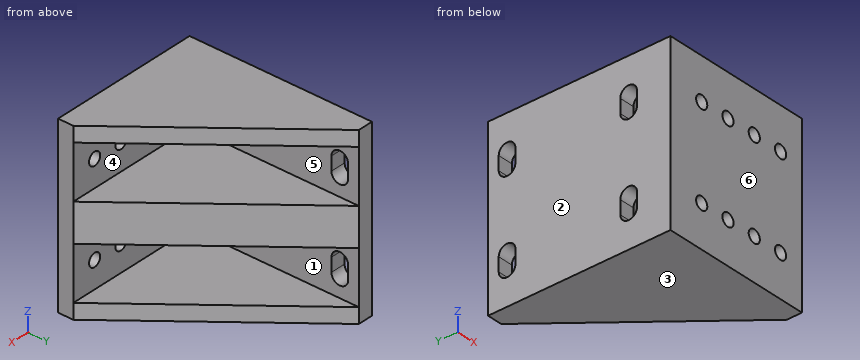
Autodesk Inventor part; units mm, degrees
ref_plane "YZ Plane" through (0, 0, 0) normal (1, 0, 0) x (0, 1, 0)
ref_plane "XZ Plane" through (0, 0, 0) normal (0, 1, 0) x (-1, 0, 0)
sketch "Sketch1" plane through (0, 0, 0) normal (0, 1, 0) x (-1, 0, 0)
  line L0 (-40, -23) -> (0, -23)
  line L1 (-40, 23) -> (0, 23)
  line L2 (0, 23) -> (0, -23)
  line L3 (-40, 23) -> (-40, -23)
  line L4 (-40, -12) -> (0, -12) construction
  line L5 (-40, 12) -> (0, 12) construction
  circle A0 centre (-9.5, 12) radius 1.7
  line L6 (-4, 23) -> (-4, -23) construction
  circle A1 centre (-17.5, 12) radius 1.7
  circle A2 centre (-25.5, 12) radius 1.7
  circle A3 centre (-33.5, 12) radius 1.7
  circle A4 centre (-9.5, -12) radius 1.7
  circle A5 centre (-17.5, -12) radius 1.7
  circle A6 centre (-25.5, -12) radius 1.7
  circle A7 centre (-33.5, -12) radius 1.7
  circle A8 centre (-9.5, 12) radius 3.5 construction
  line L7 (0, 19) -> (-40, 19) construction
  point P0 (0, 0)
  dimension "d5" = 46
  dimension "d6" = 23
  dimension "d7" = 40
  dimension "d8" = 0
  dimension "d9" = 12
  dimension "d10" = 12
  dimension "d11" = 3.4
  dimension "d12" = 4
  dimension "d13" = 9.5
  dimension "d16" = 8
  dimension "d19" = 24
  dimension "d22" = 7
  dimension "d23" = 4
extrude "Lift Attachment Plate" add sketch "Sketch1" along normal blind 4
sketch "Sketch2" plane through (0, 4, 0) normal (0, 1, 0) x (1, 0, 0)
  line L0 (0, 23) -> (0, -23)
  line L1 (40, 23) -> (0, 23)
  line L2 (0, -23) -> (4, -23)
  line L3 (4, -23) -> (4, 23)
  line L4 (4, 23) -> (0, 23)
  line L5 (0, 23) -> (0, -23)
  point P0 (0, 0)
  dimension "d26" = 4
extrude "Cross bar Attachment Plate" add sketch "Sketch2" along normal blind 44
sketch "Sketch3" plane through (0, 0, 23) normal (0, 0, 1) x (1, 0, 0)
  line L0 (4, 4) -> (4, 48)
  line L1 (4, 48) -> (4, 4)
  line L2 (40, 4) -> (4, 4)
  line L3 (4, 4) -> (40, 4)
  line L4 (40, 4) -> (4, 48)
  point P0 (0, 0)
extrude "Left bracket" add sketch "Sketch3" against normal blind 4
sketch "Sketch4" plane through (0, 0, 0) normal (0, 0, 1) x (1, 0, 0)
  line L0 (4, 48) -> (40, 4)
  line L1 (4, 4) -> (40, 4)
  line L2 (4, 48) -> (4, 4)
  line L3 (4, 4) -> (40, 4)
  line L4 (40, 4) -> (4, 48)
  point P0 (0, 0)
extrude "Center bracket" add sketch "Sketch4" along normal mid plane 10
sketch "Sketch5" plane through (40, 0, -23) normal (0, 0, -1) x (-1, 0, 0)
  line L0 (36, 48) -> (40, 48)
  line L1 (36, 48) -> (36, 4)
  line L2 (36, 48) -> (36, 4)
  line L3 (0, 4) -> (36, 4)
  line L4 (36, 4) -> (0, 4)
  line L5 (0, 4) -> (36, 48)
  point P0 (40, 0)
extrude "Right bracket" add sketch "Sketch5" against normal blind 4
sketch "Sketch6" plane through (0, 0, -23) normal (-1, 0, 0) x (0, 0, 1)
  circle A0 centre (35, 11) radius 2 construction
  circle A1 centre (11, 11) radius 2 construction
  line L0 (0, 0) -> (46, 0) construction
  line L1 (23, 57.6) -> (23, -9.6) construction
  circle A2 centre (35, 43) radius 2 construction
  circle A3 centre (11, 43) radius 2 construction
  line L2 (42, 48) -> (42, 4) construction
  line L3 (4, 4) -> (4, 48) construction
  line L4 (15, 11) -> (7, 11) construction
  line L5 (4, 4) -> (4, 48)
  line L6 (12.8, 13.2) -> (9.2, 13.2)
  line L7 (9.2, 8.8) -> (12.8, 8.8)
  arc A4 (12.8, 8.8) -> (12.8, 13.2) centre (12.8, 11) ccw
  arc A5 (9.2, 13.2) -> (9.2, 8.8) centre (9.2, 11) ccw
  point P0 (23, 0)
  dimension "d35" = 4
  dimension "d36" = 4
  dimension "d37" = 11
  dimension "d38" = 11
  dimension "d39" = 12
  dimension "d40" = 12
  dimension "d41" = 4
  dimension "d42" = 4
  dimension "d43" = 32
  dimension "d44" = 32
  dimension "d45" = 4
  dimension "d46" = 4
  dimension "d47" = 4.4
extrude "Extrusion6" cut sketch "Sketch6" against normal through all
pattern_linear "Rectangular Pattern1" count 2 spacing 24 along (0, 0, 1) count 2 spacing 32 along (0, 1, 0) of "Extrusion6"
equation "\"d38\" = d37"
equation "\"d39\" = d40"
equation "\"d44\" = d43"
equation "\"d46\" = d45"
properties part number "Cross bar bracket generic"
Could you check a few things on this model? Use its own coordinates, in mm. Face numbers are marked on the shaded views. A direction names the side the tool comes from. Coordinates: 2 decimals unless noted, no trailing zeros. Write each loop counter-clockwise with the first axis right and the second up, starting at its lowest first coordinate (ties: lowest second). Pieces come first, ordered by that corner, then holes. Notation, with made-up numbers: (20.5, 62.25) - (29.5, 62.25) arc R15 ccw to (29.5, 77.25) - close; hole circle Ø10 at (-6, 58). An arc over 180 degrees is marked (long way). Put each result on its own line as item: value. Start each with the question number.
Q1. I want a section at C-C on z = 20. Write out the boundary of the cut face in (x, y), plus the area to 3 significant figures.
Q2. Which directions (+Z, -Z, +X, -X, +Y, -Y) give clear straight access to the entire face, cutting with the end or side of a thin tool? Please do the marked faces 5 and 6.
Q3. Thinking about a two-plate mould opening in Z: for the marked faces 1, 2, 3 and 4, which applies, pulls with the +Z half, pulls with the -Z half, needs draft (parallel to the pull), parting line crosses it, or undercut?
Q4. I want a section at D-D on y = 33. Write out the boundary of the cut face in (x, z).
Q5. I'm going to push flat-ended pins straight in: P1, Ø1.8, axis at x = 2, z = 11.5, coming from the -Y side; P2, Ø4, axis at x = 33.5, z = -12, coming from the +Y side. Where does each tip first touch, or does it pass through?
Q6. Please list where these lines run through material, in increasing order: L1, parallel to Z at x = 11, y = 37; L2, parallel to Z at x = 33.5, y = 3.15; L3, parallel to Y at x = 18.5, z = -10.
Q7. I want a section at B-B on x = 3. Write out the boundary of the cut face in (y, z).
Q8. I want a section at A-A on x = 17.5. Write out the boundary of the cut face in (y, z), plus the area to 3 significant figures.
Checks:
1. outline: (0, 0) - (40, 0) - (40, 4) - (4, 48) - (0, 48) - close
1. area: 1,130 mm²
2. face 5: +X, +Y
2. face 6: +Z, -Z, +X, -X, -Y
3. face 1: undercut
3. face 2: needs draft
3. face 3: pulls with the -Z half
3. face 4: undercut
4. outline: (0, -23) - (16.27, -23) - (16.27, -19) - (4, -19) - (4, -5) - (16.27, -5) - (16.27, 5) - (4, 5) - (4, 19) - (16.27, 19) - (16.27, 23) - (0, 23) - close
5. P1: y = 0
5. P2: y = 4
6. L1: -23 to -19, -5 to 5, 19 to 23
6. L2: -23 to -13.7, -10.3 to 10.3, 13.7 to 23
6. L3: 0 to 4
7. outline: (0, -23) - (48, -23) - (48, 23) - (0, 23) - close; hole (8.8, -13.8) arc R2.2 ccw to (13.2, -13.8) - (13.2, -10.2) arc R2.2 ccw to (8.8, -10.2) - close; hole (8.8, 10.2) arc R2.2 ccw to (13.2, 10.2) - (13.2, 13.8) arc R2.2 ccw to (8.8, 13.8) - close; hole (40.8, -13.8) arc R2.2 ccw to (45.2, -13.8) - (45.2, -10.2) arc R2.2 ccw to (40.8, -10.2) - close; hole (40.8, 10.2) arc R2.2 ccw to (45.2, 10.2) - (45.2, 13.8) arc R2.2 ccw to (40.8, 13.8) - close
8. outline: (0, -23) - (31.5, -23) - (31.5, -19) - (4, -19) - (4, -13.7) - (0, -13.7) - close; (0, -10.3) - (4, -10.3) - (4, -5) - (31.5, -5) - (31.5, 5) - (4, 5) - (4, 10.3) - (0, 10.3) - close; (0, 13.7) - (4, 13.7) - (4, 19) - (31.5, 19) - (31.5, 23) - (0, 23) - close
8. area: 652 mm²
